Could you check a few things on this drawing? It's one solid part, dimensions in mm from its lowest x, y, z. A direction names the side the tool comes from. Coordinates: 2 decimals unless noted, no trailing zeros. Loops run counter-clockwise (first coordinate to the right, second up) from the corner with the lowest first, then second, coordinate; pieces in that order, holes last. Notation, with made-up numbers: (8.5, 2.25) -> (64.5, 2.25) arc R26 cw to (64.5, 18.25) -> close; hole circle Ø4 at (51.5, 9.5). An arc over 180 degrees is marked (long way). One line per question, with ' | ' between items.
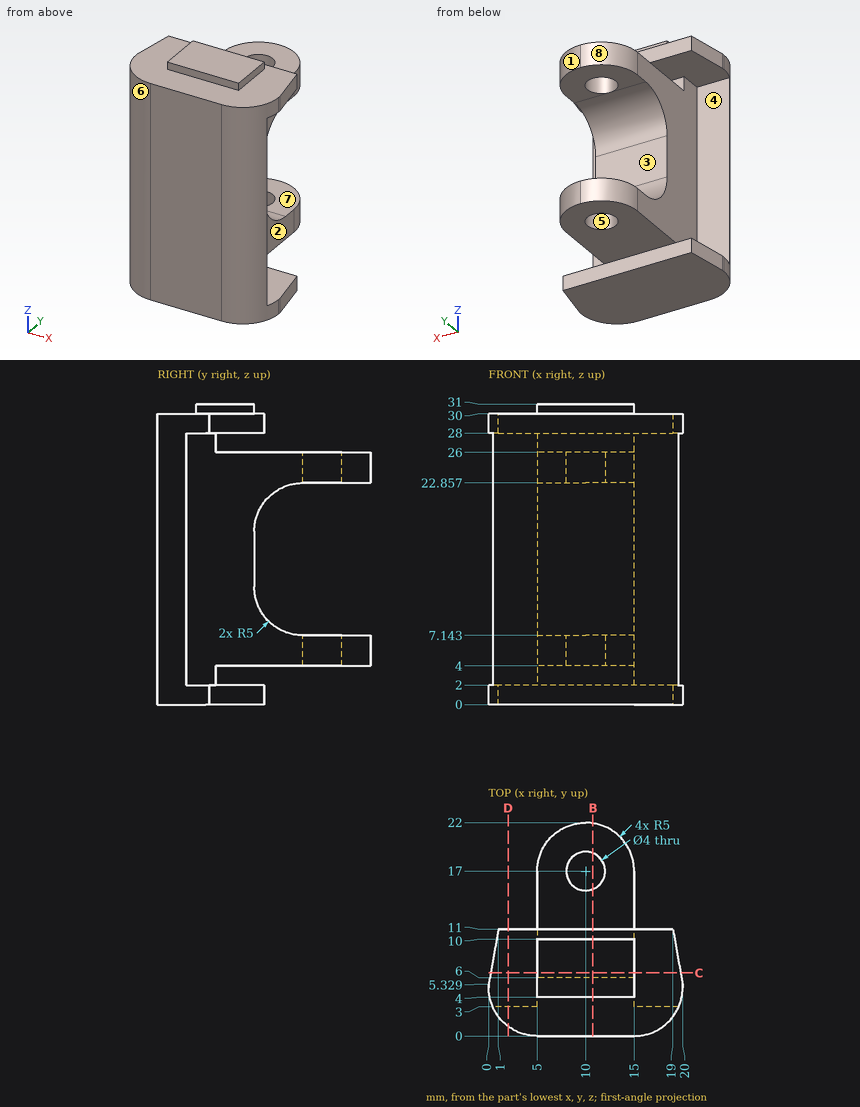
1) We'd pull the mould along Y, two halves only. Please class the marked faces 5, 6, 7 and 8: pulls with the +Y half, pulls with the -Y half, needs draft (parallel to the pull), parting line crosses it, or undercut.
Data:
face 5: undercut | face 6: pulls with the -Y half | face 7: needs draft | face 8: pulls with the +Y half
2) If we section it at C-C on y = 6.5: Please give me the cut outline in (x, z).
Data:
outline: (0.21, 0) -> (19.79, 0) -> (19.79, 2) -> (0.21, 2) -> close; (0.21, 28) -> (19.79, 28) -> (19.79, 30) -> (15, 30) -> (15, 31) -> (5, 31) -> (5, 30) -> (0.21, 30) -> close; (5, 4) -> (15, 4) -> (15, 26) -> (5, 26) -> close
3) If we section it at B-B on x = 10.75: Give the number of separate pieces and of enclosed holes in the cut face.
Data:
separate pieces: 3 | enclosed holes: 0
4) I'm going to push flat-ended pins straight in: pin 1 Ø7.5 at (x, y) = (10, 19.5) entering from +Z; pin 2 Ø0.5 at (x, z) = (12.5, 30.5) entering from -Y; pin 3 Ø0.8 at (x, z) = (9, 30.5) entering from +Y; pin 4 Ø2.5 at (x, y) = (10, 17) entering from +Z. Where does each tip first touch, or does it pass through?
Data:
pin 1: z = 26 | pin 2: y = 4 | pin 3: y = 10 | pin 4: through
5) If we section it at D-D on x = 2: Please give me the cut outline in (y, z).
Data:
outline: (1, 0) -> (11, 0) -> (11, 2) -> (3, 2) -> (3, 28) -> (11, 28) -> (11, 30) -> (1, 30) -> close
6) I need wall thicknesses on line 1 along Z through (x, y) = (5.25, 18); line 2 along Z through (x, y) = (12.5, 9.25); line 3 along Z through (x, y) = (16.5, 7.75). Which ranges of each line are inside material? Lowest first, please. Write a range as from..to.
Data:
line 1: 4..7.14, 22.86..26 | line 2: 0..2, 4..26, 28..31 | line 3: 0..2, 28..30
7) On a 3-axis mill with a long thin cutter (end or side, diameter ignored), from which of +Z, -Z, +X, -X, +Y, -Y can I reach the whole of each face in a straight line? I mean the marked faces 1, 2, 3 and 4. Say none if no direction works.
Data:
face 1: +Z, -Z, +X, +Y | face 2: +X, +Y | face 3: +X, -X, +Y | face 4: -X, +Y
